```python
from build123d import *


with BuildPart() as part:
    # Sketch1 → Revolve1 (revolve)
    with BuildSketch(Plane(origin=(0, 0, 0), x_dir=(0, 0, -1), z_dir=(1, 0, 0)), mode=Mode.PRIVATE) as revolve1_sk:
        with BuildLine():
            Line((0, 0), (0, 22.225))
            Line((0, 22.225), (105.41, 22.225))
            Line((105.41, 22.225), (105.41, 21.8186))
            Line((105.41, 21.8186), (121.412, 21.8186))
            Line((121.412, 21.8186), (121.412, 19.3675))
            ThreePointArc((121.412, 19.3675), (121.969961582, 18.020461582), (123.317, 17.4625))
            Line((123.317, 17.4625), (141.986, 17.4625))
            Line((141.986, 17.4625), (176.022, 13.4874))
            Line((176.022, 13.4874), (202.057, 13.4874))
            Line((202.057, 13.4874), (202.057, 13.2334))
            ThreePointArc((202.057, 13.2334), (202.242987194, 12.784387194), (202.692, 12.5984))
            Line((202.692, 12.5984), (204.597, 12.5984))
            Line((204.597, 12.5984), (225.8568, 12.5984))
            Line((225.8568, 12.5984), (225.8568, 0))
            Line((225.8568, 0), (0, 0))
        make_face()
    revolve(revolve1_sk.sketch.rotate(Axis((0, 0, 0), (0, 0, -1)), 90), axis=Axis((0, 0, 0), (0, 0, -1)))


solid = part.part
```
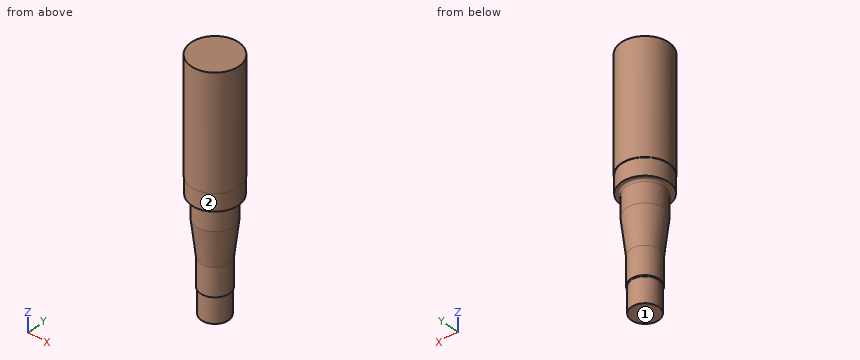
Input: part model. Units: mm. Frame: model coordinates. Face numbers are marked on the shaded views. A direction names the side the tool comes from. Give positions to 0.01 mm unless a question says otherwise; leave off trailing zeros. Order: outer loops, then holes, each group sorted by start corner. A loop starts at its lowest first (then second) coordinate and runs counter-clockwise, first axis right, second up.
1. Pin query (flat end, axial travel): pin 1 Ø3 at (y, z) = (2.5, -88) entering from -X; pin 2 Ø4 at (y, z) = (-12.5, -79) entering from -X; pin 3 Ø2 at (y, z) = (-4, -110.5) entering from -X; pin 4 Ø6 at (x, y) = (6, 12) entering from -Z. Return the tip coordinate at first contact, or that it passes through.
Computed:
pin 1: stops at x = -22.2
pin 2: stops at x = -19.59
pin 3: stops at x = -21.61
pin 4: stops at z = -225.86
2. Cut plane C-C (z = -58). Return loops of the section in (x, y) (3 decimals).
Computed:
outline: circle Ø44.45 at (0, 0)
3. Set-up query: the marked faces 1 and 2. Return all of +Z, -Z, +X, -X, +Y, -Y with unobstructed straight access to the full face (end or side cutting, diameter ignored); none if empty.
Computed:
face 1: -Z, +X, -X, +Y, -Y
face 2: -Z
4. Line query: probe 1 along Z at (x, y) = (-12, 5); probe 2 along Y at (x, z) = (-0.5, -182); probe 3 along X at (y, z) = (-7, -48). Output: solid intervals per line, ascending.
Computed:
probe 1: z = -202.1 to 0
probe 2: y = -13.48 to 13.48
probe 3: x = -21.09 to 21.09
5. Cut plane D-D (z = -156). Return loops of the section in (x, y).
Computed:
outline: circle Ø31.65 at (0, 0)
